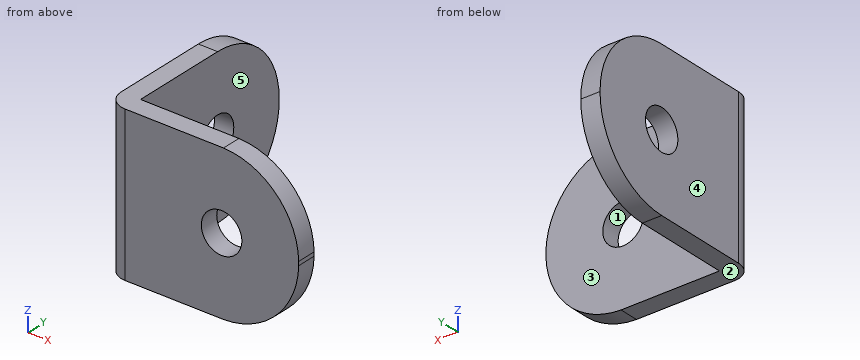
from build123d import *

# Parameters (mm, degrees)
SKETCH_1_W          = 20
SKETCH_1_H          = 20
EXTRUDE_1_DEPTH     = 16
SKETCH_2_W          = 18
SKETCH_2_H          = 18
CUT_EXTRUDE_1_DEPTH = 16
SKETCH_3_R          = 2.1
CUT_EXTRUDE_2_DEPTH = 16
SKETCH_4_R          = 2.1
CUT_EXTRUDE_3_DEPTH = 16
CUT_EXTRUDE_4_DEPTH = 16
CUT_EXTRUDE_5_DEPTH = 16
CUT_EXTRUDE_6_DEPTH = 16


with BuildPart() as part:
    # 草图1 → 凸台-拉伸1 (new body)
    with BuildSketch(Plane.XY):
        Rectangle(SKETCH_1_W, SKETCH_1_H)
    extrude(amount=EXTRUDE_1_DEPTH)

    # 草图2 → 切除-拉伸1 (cut)
    with BuildSketch(Plane.XY.offset(16)):
        with Locations((1, 1)):
            Rectangle(SKETCH_2_W, SKETCH_2_H)
    extrude(amount=-CUT_EXTRUDE_1_DEPTH, mode=Mode.SUBTRACT)

    # 草图3 → 切除-拉伸2 (cut)
    with BuildSketch(Plane(origin=(-8, 0, 0), x_dir=(0, 0, -1), z_dir=(1, 0, 0))):
        with Locations(Location((-8, 2, 0), (0, 0, 90))):
            Circle(SKETCH_3_R)
    extrude(amount=-CUT_EXTRUDE_2_DEPTH, mode=Mode.SUBTRACT)

    # 草图4 → 切除-拉伸3 (cut)
    with BuildSketch(Plane(origin=(0, -8, 0), x_dir=(1, 0, 0), z_dir=(0, 1, 0))):
        with Locations(Location((2, -8, 0), (0, 0, 180))):
            Circle(SKETCH_4_R)
    extrude(amount=-CUT_EXTRUDE_3_DEPTH, mode=Mode.SUBTRACT)

    # 草图5 → 切除-拉伸4 (cut)
    with BuildSketch(Plane(origin=(-8, 0, 0), x_dir=(0, 0, -1), z_dir=(1, 0, 0))):
        with BuildLine():
            Line((-16, 10), (-16, 2))
            ThreePointArc((-16, 2), (-13.656854261, 7.656854238), (-8.000000031, 10))
            Line((-8.000000031, 10), (-16, 10))
        make_face()
        with BuildLine():
            Line((0, 10), (-8.000000031, 10))
            ThreePointArc((-8.000000031, 10), (-2.343145762, 7.656854261), (0, 2))
            Line((0, 2), (0, 10))
        make_face()
    extrude(amount=-CUT_EXTRUDE_4_DEPTH, mode=Mode.SUBTRACT)

    # 草图6 → 切除-拉伸5 (cut)
    with BuildSketch(Plane(origin=(0, -8, 0), x_dir=(1, 0, 0), z_dir=(0, 1, 0))):
        with BuildLine():
            Line((10, -7.79882112), (10, 0))
            Line((10, 0), (2.20117888, 0))
            ThreePointArc((2.20117888, 0), (7.658642635, -2.341357365), (10, -7.79882112))
        make_face()
        with BuildLine():
            Line((10, -16), (10, -8.20117888))
            ThreePointArc((10, -8.20117888), (7.658642635, -13.658642635), (2.20117888, -16))
            Line((2.20117888, -16), (10, -16))
        make_face()
    extrude(amount=-CUT_EXTRUDE_5_DEPTH, mode=Mode.SUBTRACT)

    # 草图7 → 切除-拉伸6 (cut)
    with BuildSketch(Plane.XY.offset(16)):
        with BuildLine():
            Line((-10, -8), (-10, -10))
            Line((-10, -10), (-8, -10))
            ThreePointArc((-8, -10), (-9.414213562, -9.414213562), (-10, -8))
        make_face()
    extrude(amount=-CUT_EXTRUDE_6_DEPTH, mode=Mode.SUBTRACT)


solid = part.part
The model under review builds one solid part; all positions refer to its coordinate system, in mm. Face numbers are marked on the shaded views. A direction names the side the tool comes from. Coordinates: 2 decimals unless noted, no trailing zeros. Write each loop counter-clockwise with the first axis right and the second up, starting at its lowest first coordinate (ties: lowest second). Pieces come first, ordered by that corner, then holes. Notation, with made-up numbers: (69.5, -20.75) - (89.5, -20.75) arc R35 ccw to (89.5, 12.25) - close; hole circle Ø9 at (12.25, 17). An arc over 180 degrees is marked (long way). Answer as a JSON object with one key per item and string values. Group by question number.
1. Add section B-B (x = 3.25). Give the boundary of the cut face in (y, z), plus the area to 3 significant figures.
2. To check wall thickness, follow probe 1 along Z at (x, y) = (-8.45, 2); probe 2 along Y at (x, z) = (-4.75, 3.25). State the ranges of each line that lie inside material, in increasing order.
3. Clearance check with flat-ended pins moving along their axes: pin 1 Ø5 at (y, z) = (4.5, 11.5) entering from +X; pin 2 Ø8 at (x, z) = (-1.5, 9) entering from +Y. State where each tip first meets the part, or that it passes through.
4. Mouldability with a two-part tool opening along Z and no side actions: class the marked faces 1, 2 and 3 as pulls with the +Z half, pulls with the -Z half, needs draft (parallel to the pull), parting line crosses it, or undercut.
5. Add section D-D (z = 14.75). Give the boundary of the cut face in (x, y), plus the area to 3 significant figures.
6. Add section C-C (y = -6.75). Give the boundary of the cut face in (x, z).
7. Machinability: for the marked faces 4 and 5, which of the approach directions +Z, -Z, +X, -X, +Y, -Y give a long, thin tool a straight path to every point of the face, cutting with its end or side? Answer none if there is none.
8. Add section A-A (z = 8.5). Give the boundary of the cut face in (x, y), plus the area to 3 significant figures.
Findings:
{
 "1": {"outline": "(-10, 0.1) - (-8, 0.1) - (-8, 6.31) - (-10, 6.31) - close; (-10, 9.69) - (-8, 9.69) - (-8, 15.9) - (-10, 15.9) - close", "area": "24.9 mm²"},
 "2": {"probe 1": "0 to 5.9, 10.1 to 16", "probe 2": "-10 to -8"},
 "3": {"pin 1": "x = -8", "pin 2": "y = -8"},
 "4": {"face 1": "undercut", "face 2": "pulls with the -Z half", "face 3": "needs draft"},
 "5": {"outline": "(-10, -8) arc R2 ccw to (-8, -10) - (6.3, -10) - (6.3, -8) - (-8, -8) - (-8, 6.29) - (-10, 6.29) - close", "area": "60.3 mm²"},
 "6": {"outline": "(-10, 0) - (-8, 0) - (-8, 16) - (-10, 16) - close"},
 "7": {"face 4": "+Z, -Z, -X, +Y, -Y", "face 5": "+Z, -Z, +X, +Y"},
 "8": {"outline": "(-10, -8) arc R2 ccw to (-8, -10) - (-0.04, -10) - (-0.04, -8) - (-8, -8) - (-8, -0.04) - (-10, -0.04) - close; (-10, 4.04) - (-8, 4.04) - (-8, 9.98) - (-10, 9.98) - close; (4.04, -10) - (9.99, -10) - (9.99, -8) - (4.04, -8) - close", "area": "58.8 mm²"}
}
